The model under review builds one solid part; all positions refer to its coordinate system, in mm. A direction names the side the tool comes from. Round coordinates to 2 decimals unless told otherwise and drop trailing zeros. Write each loop counter-clockwise with the first axis right and the second up, starting at its lowest first coordinate (ties: lowest second). Pieces come first, ordered by that corner, then holes. Notation, with made-up numbers: M 58,-24.5 L 76,-24.5 A10 ccw 76,-19.5 Z; hole C 65.25,7 d8. An arc over 180 degrees is marked long. Write item = value, one per line. Start each with the question number.
Item 1: For pin 1 Ø4 at (x, y) = (16.5, 6.5) entering from -Z; pin 2 Ø9.5 at (x, z) = (-5, 7) entering from +Y; pin 3 Ø5 at (x, y) = (-14, -14.5) entering from +Z, all flat-tipped, find the tip position at first contact; note any pin that passes through.
Item 2: Take a section at A-A, the plane y = -8.5. Give the boundary of the cut face in (x, z), plus the area to 3 significant figures.
Item 3: To check wall thickness, follow line 1 along Z through (x, y) = (21.5, -14). State the ranges of the line that lie inside material, in increasing order.
Item 4: The part is to be moulded in two halves that separate along X. For faces 1 (the flat face through (0, -18.13, 6)), 2 (the flat face through (0, -18.13, 238)), 3 (the flat face through (34, 0, 120)), 4 (the flat face through (0, 19.4, 148)), say which applies: +X half, -X half, draft (parallel to the pull), parting line (faces both ways), or undercut.
Item 5: Tool access review of faces 5 (the flat face through (-32.73, 1, 6)), 6 (the flat face through (-32.73, 1, 238)), 7 (the flat face through (0, -19.4, 120)): name each direction out of +Z, -Z, +X, -X, +Y, -Y from which nothing blocks a thin tool from reaching the whole face with its end or side.
Item 6: Take a section at B-B, the plane x = 21.5. Give the boundary of the cut face in (y, z), plus the area to 3 significant figures.
Autodesk Inventor part; units mm, degrees
ref_plane "Work Plane1" through (34, -18.13, 0) normal (0, -1, 0) x (1, 0, 0)
ref_plane "YZ Plane" through (0, 0, 0) normal (1, 0, 0) x (0, 1, 0)
ref_plane "XZ Plane" through (0, 0, 0) normal (0, 1, 0) x (-1, 0, 0)
sketch "Sketch1" plane through (0, 0, 0) normal (0, 0, 1) x (1, 0, 0)
  line L0 (-34, -19.4) -> (34, -19.4)
  line L1 (34, -19.4) -> (34, 19.4)
  line L2 (34, 19.4) -> (-34, 19.4)
  line L3 (-34, 19.4) -> (-34, -19.4)
  line L4 (-34, -19.4) -> (34, 19.4) construction
  line L5 (34, -19.4) -> (-34, 19.4) construction
  point P0 (0, 0)
  dimension "d0" = 68
  dimension "d1" = 38.8
extrude "Extrusion1" add sketch "Sketch1" along normal blind 244.2
sketch "Sketch2" plane through (-34, 19.4, 0) normal (0, 1, 0) x (1, 0, 0)
  line L0 (68, -244.2) -> (0, -244.2)
  line L1 (68, 0) -> (0, 0)
  arc A0 (19.15, -236.7) -> (14.65, -236.7) centre (16.9, -236.7) ccw
  arc A1 (53.35, -236.7) -> (48.85, -236.7) centre (51.1, -236.7) ccw
  arc A2 (48.85, -7.5) -> (53.35, -7.5) centre (51.1, -7.5) ccw
  arc A3 (14.65, -7.5) -> (19.15, -7.5) centre (16.9, -7.5) ccw
  line L2 (16.9, -236.7) -> (16.9, -7.5) construction
  line L3 (16.9, -7.5) -> (51.1, -7.5) construction
  line L4 (51.1, -7.5) -> (51.1, -236.7) construction
  line L5 (16.9, -236.7) -> (16.9, -244.2) construction
  line L6 (16.9, -7.5) -> (16.9, 0) construction
  line L7 (16.9, -7.5) -> (0, 0) construction
  line L8 (51.1, -7.5) -> (68, 0) construction
  line L9 (48.85, -236.7) -> (48.85, -244.2)
  line L10 (53.35, -236.7) -> (53.35, -244.2)
  line L11 (14.65, -236.7) -> (14.65, -244.2)
  line L12 (19.15, -236.7) -> (19.15, -244.2)
  line L13 (19.15, -7.5) -> (19.15, 0)
  line L14 (14.65, -7.5) -> (14.65, 0)
  line L15 (53.35, -7.5) -> (53.35, 0)
  line L16 (48.85, -7.5) -> (48.85, 0)
  point P0 (34, 0)
  dimension "d4" = 2.25
  dimension "d5" = 229.2
  dimension "d6" = 34.2
extrude "Extrusion2" cut sketch "Sketch2" against normal up to surface (38.8 mm away)
ref_plane "Work Plane1" through (34, -18.13, 0) normal (0, -1, 0) x (1, 0, 0)
sketch "Sketch3" plane through (-34, 19.4, 244.2) normal (0, 1, 0) x (1, 0, 0)
  line L0 (0, 244.2) -> (0, 0)
  line L1 (68, 244.2) -> (68, 0)
  line L2 (66.73, 0) -> (66.73, 12)
  line L3 (66.73, 12) -> (1.27, 12)
  line L4 (1.27, 12) -> (1.27, 0)
  line L5 (1.27, 0) -> (66.73, 0)
  line L6 (1.27, 0) -> (0, 0) construction
  line L7 (68, 0) -> (66.73, 0) construction
  line L8 (1.27, 232.2) -> (66.73, 232.2)
  line L9 (66.73, 232.2) -> (66.73, 244.2)
  line L10 (66.73, 244.2) -> (1.27, 244.2)
  line L11 (1.27, 244.2) -> (1.27, 232.2)
  line L12 (1.27, 244.2) -> (0, 244.2) construction
  point P0 (34, 244.2)
  dimension "d9" = 1.27
  dimension "d14" = 220.2
extrude "Extrusion3" cut sketch "Sketch3" against normal up to surface (37.53 mm away)
properties part number "UHP-1500-230"
Response values:
q1.pin_1 = 12
q1.pin_2 = -18.13
q1.pin_3 = 232.2
q2.outline = M -34,0 L -32.73,0 L -32.73,12 L 32.73,12 L 32.73,0 L 34,0 L 34,244.2 L 32.73,244.2 L 32.73,232.2 L -32.73,232.2 L -32.73,244.2 L -34,244.2 Z
q2.area = 15,000 mm2
q3.line_1 = 12 to 232.2
q4.face_1 = undercut
q4.face_2 = undercut
q4.face_3 = +X half
q4.face_4 = draft
q5.face_5 = -Z, +Y
q5.face_6 = +Z, +Y
q5.face_7 = +Z, -Z, +X, -X, -Y
q6.outline = M -19.4,0 L -18.13,0 L -18.13,12 L 19.4,12 L 19.4,232.2 L -18.13,232.2 L -18.13,244.2 L -19.4,244.2 Z
q6.area = 8,570 mm2
